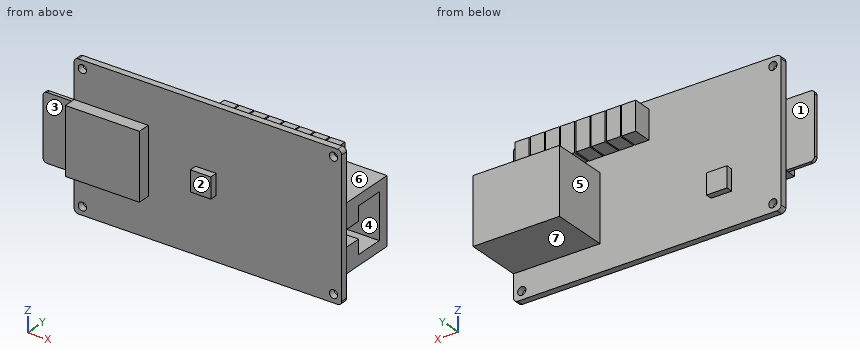
from build123d import *

# Parameters (mm, degrees)
SKIZZE1_W                       = 65
SKIZZE1_H                       = 35
SKIZZE1_R                       = 1
AUFSATZ_LINEAR_AUSTRAGEN1_DEPTH = 1.6
VERRUNDUNG1_R                   = 1
SKIZZE2_W                       = 18
SKIZZE2_H                       = 16
AUFSATZ_LINEAR_AUSTRAGEN2_DEPTH = 3
SKIZZE3_W                       = 15.998
SKIZZE3_H                       = 0.8
AUFSATZ_LINEAR_AUSTRAGEN3_DEPTH = 7
VERRUNDUNG2_R                   = 1
SKIZZE4_W                       = 21
SKIZZE4_H                       = 16
AUFSATZ_LINEAR_AUSTRAGEN4_DEPTH = 13.7
SCHNITT_LINEAR_AUSTRAGEN1_DEPTH = 12
SKIZZE6_W                       = 3.4
SKIZZE6_H                       = 7
AUFSATZ_LINEAR_AUSTRAGEN5_DEPTH = 4.5
SKIZZE7_W                       = 5
SKIZZE7_H                       = 5
AUFSATZ_LINEAR_AUSTRAGEN6_DEPTH = 1.8
SKIZZE8_W                       = 5
SKIZZE8_H                       = 5
AUFSATZ_LINEAR_AUSTRAGEN7_DEPTH = 1.6


with BuildPart() as part:
    # Skizze1 → Aufsatz-Linear austragen1 (new body)
    with BuildSketch(Plane(origin=(0, 0, 0), x_dir=(1, 0, 0), z_dir=(0, 1, 0))):
        Rectangle(SKIZZE1_W, SKIZZE1_H)
        with Locations((-30.5, -15.5)):
            Circle(SKIZZE1_R, mode=Mode.SUBTRACT)
        with Locations((30.5, -15.5)):
            Circle(SKIZZE1_R, mode=Mode.SUBTRACT)
        with Locations((30.5, 15.5)):
            Circle(SKIZZE1_R, mode=Mode.SUBTRACT)
        with Locations((-30.5, 15.5)):
            Circle(SKIZZE1_R, mode=Mode.SUBTRACT)
    extrude(amount=AUFSATZ_LINEAR_AUSTRAGEN1_DEPTH)

    # Verrundung1
    verrundung1_edges = [part.edges().sort_by_distance(p)[0] for p in [
        (32.5, 0.8, -17.5),
        (32.5, 0.8, 17.5),
        (-32.5, 0.8, 17.5),
        (-32.5, 0.8, -17.5),
    ]]
    fillet(verrundung1_edges, radius=VERRUNDUNG1_R)

    # Skizze2 → Aufsatz-Linear austragen2 (add)
    with BuildSketch(Plane.XZ):
        with Locations((-23.49, 0)):
            Rectangle(SKIZZE2_W, SKIZZE2_H)
    extrude(amount=AUFSATZ_LINEAR_AUSTRAGEN2_DEPTH)

    # Skizze3 → Aufsatz-Linear austragen3 (add)
    with BuildSketch(Plane.ZY.offset(32.49)):
        with Locations((0, -0.401)):
            Rectangle(SKIZZE3_W, SKIZZE3_H)
    extrude(amount=AUFSATZ_LINEAR_AUSTRAGEN3_DEPTH)

    # Verrundung2
    verrundung2_edges = [part.edges().sort_by_distance(p)[0] for p in [
        (-39.49, -0.401, -7.999),
        (-39.49, -0.401, 7.999),
    ]]
    fillet(verrundung2_edges, radius=VERRUNDUNG2_R)

    # Skizze4 → Aufsatz-Linear austragen4 (add)
    with BuildSketch(Plane(origin=(0, 1.6, 0), x_dir=(1, 0, 0), z_dir=(0, 1, 0))):
        with Locations((21.999, 3)):
            Rectangle(SKIZZE4_W, SKIZZE4_H)
    extrude(amount=AUFSATZ_LINEAR_AUSTRAGEN4_DEPTH)

    # Skizze5 → Schnitt-Linear austragen1 (cut)
    with BuildSketch(Plane(origin=(32.499, 0, 0), x_dir=(0, 0, -1), z_dir=(1, 0, 0))):
        Polygon((8.5, 12.7), (-2.5, 12.7), (-2.5, 5.7), (1, 5.7), (1, 1.7), (5, 1.7), (5, 5.7), (8.5, 5.7), align=None)
    extrude(amount=-SCHNITT_LINEAR_AUSTRAGEN1_DEPTH, mode=Mode.SUBTRACT)

    # Skizze6 → Aufsatz-Linear austragen5 (add)
    with BuildSketch(Plane(origin=(0, 1.6, 0), x_dir=(1, 0, 0), z_dir=(0, 1, 0))):
        with Locations((27.2, -12)):
            Rectangle(SKIZZE6_W, SKIZZE6_H)
        with Locations((23.5, -12)):
            Rectangle(SKIZZE6_W, SKIZZE6_H)
        with Locations((19.8, -12)):
            Rectangle(SKIZZE6_W, SKIZZE6_H)
        with Locations((16.1, -12)):
            Rectangle(SKIZZE6_W, SKIZZE6_H)
        with Locations((12.4, -12)):
            Rectangle(SKIZZE6_W, SKIZZE6_H)
        with Locations((8.7, -12)):
            Rectangle(SKIZZE6_W, SKIZZE6_H)
        with Locations((5, -12)):
            Rectangle(SKIZZE6_W, SKIZZE6_H)
        with Locations((1.3, -12)):
            Rectangle(SKIZZE6_W, SKIZZE6_H)
    extrude(amount=AUFSATZ_LINEAR_AUSTRAGEN5_DEPTH)

    # Skizze7 → Aufsatz-Linear austragen6 (add)
    with BuildSketch(Plane.XZ):
        with Locations((-0.5, 0)):
            Rectangle(SKIZZE7_W, SKIZZE7_H)
    extrude(amount=AUFSATZ_LINEAR_AUSTRAGEN6_DEPTH)

    # Skizze8 → Aufsatz-Linear austragen7 (add)
    with BuildSketch(Plane(origin=(0, 1.6, 0), x_dir=(1, 0, 0), z_dir=(0, 1, 0))):
        with Locations((-18, 7)):
            Rectangle(SKIZZE8_W, SKIZZE8_H)
    extrude(amount=AUFSATZ_LINEAR_AUSTRAGEN7_DEPTH)


solid = part.part
Read the model definition and answer for the solid it produces. Units are mm, in the model's axes. Face numbers are marked on the shaded views. A direction names the side the tool comes from. Coordinates: 2 decimals unless noted, no trailing zeros. Order: outer loops, then holes, each group sorted by start corner. A loop starts at its lowest first (then second) coordinate and runs counter-clockwise, first axis right, second up. Notation, with made-up numbers: (18.25, 14) - (53.25, 14) arc R17 cw to (53.25, 27) - close; hole circle Ø3 at (71, 83.25). An arc over 180 degrees is marked (long way). Use one line per item in the form item = value.
(1) Section B-B, the plane z = -15.5 is taken. Give the vertices of the cut face in (x, y).
Computed values:
outline = (-32.5, 0) - (-31.5, 0) - (-31.5, 1.6) - (-32.5, 1.6) - close; (-29.5, 0) - (29.5, 0) - (29.5, 1.6) - (-29.5, 1.6) - close; (31.5, 0) - (32.5, 0) - (32.5, 1.6) - (31.5, 1.6) - close
(2) Section C-C, the plane x = -30.5 is taken. Give the vertices of the cut face in (y, z).
Computed values:
outline = (-3, -8) - (0, -8) - (0, -14.5) - (1.6, -14.5) - (1.6, 14.5) - (0, 14.5) - (0, 8) - (-3, 8) - close; (0, -17.5) - (1.6, -17.5) - (1.6, -16.5) - (0, -16.5) - close; (0, 16.5) - (1.6, 16.5) - (1.6, 17.5) - (0, 17.5) - close
(3) Straight lines are drawn through the part: L1, parallel to Z at x = 30.5, y = 0.5; L2, parallel to X at y = 0.7, z = 15.5; L3, parallel to Z at x = 29, y = 7.75. For each, find the intervals that lie inside material, in ascending order.
Computed values:
L1 = -17.5 to -16.5, -14.5 to 14.5, 16.5 to 17.5
L2 = -32.5 to -31.5, -29.5 to 29.5, 31.5 to 32.5
L3 = -11 to -8.5, 2.5 to 5
(4) Section A-A, the plane x = 30.5 is taken. Give the vertices of the cut face in (y, z).
Computed values:
outline = (0, -17.5) - (1.6, -17.5) - (1.6, -16.5) - (0, -16.5) - close; (0, -14.5) - (1.6, -14.5) - (1.6, -11) - (15.3, -11) - (15.3, 5) - (1.6, 5) - (1.6, 14.5) - (0, 14.5) - close; (0, 16.5) - (1.6, 16.5) - (1.6, 17.5) - (0, 17.5) - close; hole (1.7, -5) - (5.7, -5) - (5.7, -8.5) - (12.7, -8.5) - (12.7, 2.5) - (5.7, 2.5) - (5.7, -1) - (1.7, -1) - close
(5) Section D-D, the plane y = 4 is taken. Give the number of separate pieces and of enclosed holes in the cut face, then the cut area to 3 significant figures.
Computed values:
separate_pieces = 9
enclosed_holes = 0
area = 478 mm²
(6) Given pin 1 Ø1.7 at (x, z) = (19.5, 12) entering from +Y; pin 2 Ø5 at (y, z) = (10.5, -2.5) entering from -X; pin 3 Ø1.3 at (y, z) = (5, 12.5) entering from +X, each flat-ended and moving along its own axis, determine where each tip first touches the part or whether it passes through.
Computed values:
pin_1 = 6.1
pin_2 = 11.5
pin_3 = 28.9
(7) Which of the six approach directions +Z, -Z, +X, -X, +Y, -Y give full straight-line access (tool end or side, diameter ignored) to the marked faces 1, 2 and 3?
Computed values:
face_1 = +Z, -Z, -X, +Y
face_2 = +Z, -Z, +X, -Y
face_3 = +Z, -Z, -X, -Y
(8) For a pull along Z with two mould halves and no side action, classify the marked faces 4, 5, 6 and 7 as pulls with the +Z half, pulls with the -Z half, needs draft (parallel to the pull), parting line crosses it, or undercut.
Computed values:
face_4 = undercut
face_5 = needs draft
face_6 = undercut
face_7 = pulls with the -Z half
